from build123d import *

# Parameters (mm, degrees)
F1_DEPTH = 269.24
F2_W     = 14.478
F2_H     = 25.908
F3_DEPTH = 25.4


with BuildPart() as f1:
    # F0 (on Right) → F1 (new body)
    with BuildSketch(Plane.YZ):
        Polygon((0, 3.302), (0, 0), (71.1500963645, 19.0646108623), (142.3001927289, 0), (142.3001927289, 3.302), (71.1500963645, 22.3666108623), align=None)
    extrude(amount=-F1_DEPTH)

    # F2 (on face) → F3 (cut)
    with BuildSketch(Plane(origin=(0, -0.8255, 3.0808079416), x_dir=(1, 0, 0), z_dir=(0, -0.2588190451, 0.9659258263))):
        with Locations((-232.029, 55.4646204869)):
            Rectangle(F2_W, F2_H)
        with Locations((-232.029, 29.0486204869)):
            Rectangle(F2_W, F2_H)
        with Locations((-217.043, 55.4646204869)):
            Rectangle(F2_W, F2_H)
        with Locations((-217.043, 29.0486204869)):
            Rectangle(F2_W, F2_H)
        with Locations((-202.057, 55.4646204869)):
            Rectangle(F2_W, F2_H)
        with Locations((-202.057, 29.0486204869)):
            Rectangle(F2_W, F2_H)
        with Locations((-187.071, 55.4646204869)):
            Rectangle(F2_W, F2_H)
        with Locations((-187.071, 29.0486204869)):
            Rectangle(F2_W, F2_H)
        with Locations((-172.085, 55.4646204869)):
            Rectangle(F2_W, F2_H)
        with Locations((-172.085, 29.0486204869)):
            Rectangle(F2_W, F2_H)
        with Locations((-157.099, 55.4646204869)):
            Rectangle(F2_W, F2_H)
        with Locations((-157.099, 29.0486204869)):
            Rectangle(F2_W, F2_H)
        with Locations((-142.113, 55.4646204869)):
            Rectangle(F2_W, F2_H)
        with Locations((-142.113, 29.0486204869)):
            Rectangle(F2_W, F2_H)
        with Locations((-127.127, 55.4646204869)):
            Rectangle(F2_W, F2_H)
        with Locations((-127.127, 29.0486204869)):
            Rectangle(F2_W, F2_H)
        with Locations((-112.141, 55.4646204869)):
            Rectangle(F2_W, F2_H)
        with Locations((-112.141, 29.0486204869)):
            Rectangle(F2_W, F2_H)
        with Locations((-97.155, 55.4646204869)):
            Rectangle(F2_W, F2_H)
        with Locations((-97.155, 29.0486204869)):
            Rectangle(F2_W, F2_H)
        with Locations((-82.169, 55.4646204869)):
            Rectangle(F2_W, F2_H)
        with Locations((-82.169, 29.0486204869)):
            Rectangle(F2_W, F2_H)
        with Locations((-67.183, 55.4646204869)):
            Rectangle(F2_W, F2_H)
        with Locations((-67.183, 29.0486204869)):
            Rectangle(F2_W, F2_H)
        with Locations((-52.197, 55.4646204869)):
            Rectangle(F2_W, F2_H)
        with Locations((-52.197, 29.0486204869)):
            Rectangle(F2_W, F2_H)
        with Locations((-37.211, 55.4646204869)):
            Rectangle(F2_W, F2_H)
        with Locations((-37.211, 29.0486204869)):
            Rectangle(F2_W, F2_H)
    extrude(amount=-F3_DEPTH, mode=Mode.SUBTRACT)


solid = f1.part
Source: CAD feature listing. Evaluate the final solid. Frame: model axes, mm. Give positions to 0.01 mm unless a question says otherwise; leave off trailing zeros. Write each loop counter-clockwise with the first axis right and the second up, starting at its lowest first coordinate (ties: lowest second). Pieces come first, ordered by that corner, then holes. Notation, with made-up numbers: M 89,16.25 L 101,16.25 A20 ccw 101,46.25 Z; hole C 82.25,-5 d4. An arc over 180 degrees is marked long. Return JSON: item names as keys, results as strings. Group by question number.
1) Material intervals for line 1 along Z through (x, y) = (-223, 73.5); line 2 along Z through (x, y) = (-16, 100), sorted ascending. Write a range as [from, to].
2) Pin query (flat end, axial travel): P1, Ø12, axis at x = -203.5, y = 76, coming from the -Z side; P2, Ø6, axis at x = -77, y = 84, coming from the -Z side; P3, Ø10, axis at y = 106, z = 4, coming from the -X side; P4, Ø10, axis at x = -114.5, y = 59, coming from the +Z side. Return the tip coordinate at first contact, or that it passes through.
3) Pull-direction query (X, two-part tool) for faces 1 (the face through (-29.972, 27, 9)), 2 (the face through (-132.735, 12.356, 6.613)), 3 (the face through (0, 71, 20)); classes: pulls with the +X half, pulls with the -X half, needs draft (parallel to the pull), parting line crosses it, or undercut.
4) Cut plane C-C, the plane y = 50. Give the number of separate pieces and of enclosed holes in the cut face, plus the area to 3 significant figures.
5) Cut plane B-B, the plane y = 89.5. Output: boundary loops of the cut face in (x, z).
6) Cut plane A-A, the plane x = -115. Output: boundary loops of the cut face in (y, z).
Recorded:
{
 "1": {"line 1": "z = [18.43, 21.74]", "line 2": "z = [11.33, 14.64]"},
 "2": {"P1": "stops at z = 16.16", "P2": "stops at z = 14.82", "P3": "passes through", "P4": "stops at z = 19.4"},
 "3": {"face 1": "undercut", "face 2": "needs draft", "face 3": "pulls with the +X half"},
 "4": {"separate pieces": "15", "enclosed holes": "0", "area": "220 mm²"},
 "5": {"outline": "M -269.24,14.15 L 0,14.15 L 0,17.45 L -269.24,17.45 Z"},
 "6": {"outline": "M 0,0 L 15.55,4.17 L 14.72,7.25 L 0,3.3 Z; M 39.75,13.95 L 40.57,10.87 L 41.06,11 L 40.24,14.08 Z; M 65.26,20.79 L 66.09,17.71 L 71.15,19.06 L 142.3,0 L 142.3,3.3 L 71.15,22.37 Z"}
}
